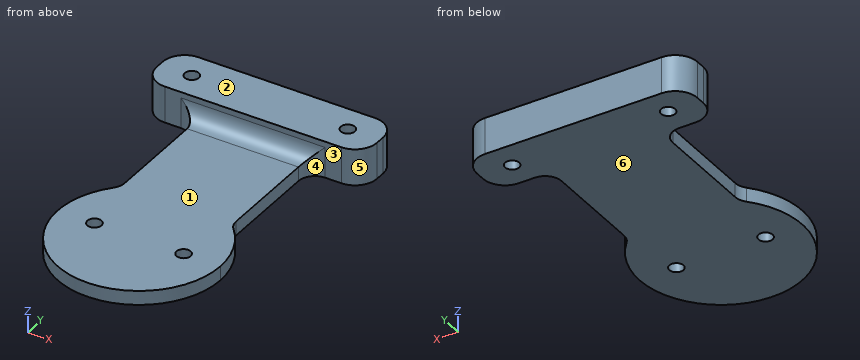
```python
from build123d import *

# Parameters (mm, degrees)
F1_DEPTH = 3.175
F3_DEPTH = 5
F4_R     = 3.6792614691
F5_R     = 1.5875
F6_DEPTH = 24.13
F7_DEPTH = 25.4
F8_R     = 4.9056819587


with BuildPart() as f1:
    # F0 (on Top) → F1 (new body)
    with BuildSketch(Plane.XY):
        with BuildLine():
            ThreePointArc((-12.4973059814, 13.2996181602), (0, 18.25), (12.4973059814, 13.2996181602))
            Line((12.4973059814, 13.2996181602), (12.4973059814, 40.75))
            Line((12.4973059814, 40.75), (24.7193473562, 40.75))
            Line((24.7193473562, 40.75), (24.7193473562, 52.75))
            Line((24.7193473562, 52.75), (-24.7193473562, 52.75))
            Line((-24.7193473562, 52.75), (-24.7193473562, 40.75))
            Line((-24.7193473562, 40.75), (-12.4973059814, 40.75))
            Line((-12.4973059814, 40.75), (-12.4973059814, 13.2996181602))
        make_face()
        with BuildLine():
            ThreePointArc((-12.4973059814, 13.2996181602), (-7.2452282862, -16.7501990161), (18.25, 0))
            ThreePointArc((18.25, 0), (16.7501990161, 7.2452282862), (12.4973059814, 13.2996181602))
            ThreePointArc((12.4973059814, 13.2996181602), (0, 18.25), (-12.4973059814, 13.2996181602))
        make_face()
    extrude(amount=F1_DEPTH)

    # F2 (on face) → F3 (join)
    with BuildSketch(Plane.XY.offset(3.175)):
        Polygon((-24.7193473562, 40.75), (-12.4973059814, 40.75), (12.4973059814, 40.75), (24.7193473562, 40.75), (24.7193473562, 52.75), (-24.7193473562, 52.75), align=None)
    extrude(amount=F3_DEPTH)

    # F4
    f4_edges = [f1.edges().sort_by_distance(p)[0] for p in [
        (12.497306, 13.299618, 1.5875),
        (-12.497306, 13.299618, 1.5875),
        (12.497306, 40.75, 1.5875),
        (0, 40.75, 3.175),
        (-12.497306, 40.75, 1.5875),
    ]]
    fillet(f4_edges, radius=F4_R)

    # F5 (on face) → F6 (cut)
    with BuildSketch(Plane.XY.offset(3.175)):
        with Locations((-10, 0)):
            Circle(F5_R)
        with Locations((10, 0)):
            Circle(F5_R)
        with Locations((17.5, 46.75)):
            Circle(F5_R)
        with Locations((-17.5, 46.75)):
            Circle(F5_R)
    extrude(amount=F6_DEPTH, mode=Mode.SUBTRACT)

    # F5 (on face) → F7 (cut)
    with BuildSketch(Plane.XY.offset(3.175)):
        with Locations((-10, 0)):
            Circle(F5_R)
        with Locations((10, 0)):
            Circle(F5_R)
        with Locations((17.5, 46.75)):
            Circle(F5_R)
        with Locations((-17.5, 46.75)):
            Circle(F5_R)
    extrude(amount=-F7_DEPTH, mode=Mode.SUBTRACT)

    # F8
    f8_edges = [f1.edges().sort_by_distance(p)[0] for p in [
        (24.719347, 40.75, 4.0875),
        (24.719347, 52.75, 4.0875),
        (-24.719347, 52.75, 4.0875),
        (-24.719347, 40.75, 4.0875),
    ]]
    fillet(f8_edges, radius=F8_R)


solid = f1.part
```
Could you check a few things on this model? Use its own coordinates, in mm. Face numbers are marked on the shaded views. A direction names the side the tool comes from. Round coordinates to 2 decimals unless told otherwise and drop trailing zeros. Loops run counter-clockwise (first coordinate to the right, second up) from the corner with the lowest first, then second, coordinate; pieces in that order, holes last. Notation, with made-up numbers: (3, 88) -> (30, 88) arc R10 ccw to (30, 107) -> close; hole circle Ø8 at (86.5, 24). An arc over 180 degrees is marked (long way). One line per question, with ' | ' between items.
(1) If we section it at A-A on z = 1: Count the separate pieces of the cut face and the enclosed holes in it, and give its area (3 significant figures).
Model answer:
separate pieces: 1 | enclosed holes: 4 | area: 2,190 mm^2
(2) For pin 1 Ø2 at (x, y) = (11.5, 31) entering from +Z (3 decimals); pin 2 Ø4 at (x, y) = (15, 23.5) entering from -Z; pin 3 Ø1 at (y, z) = (9, 3.5) entering from -X; pin 4 Ø1.6 at (y, z) = (26.5, 1) entering from -X, each with a flat end and sliding along its axis, tell me the tip position at first contact or that it passes through.
Model answer:
pin 1: stops at z = 3.175 | pin 2: passes through | pin 3: stops at x = -16.09 | pin 4: stops at x = -12.5
(3) If we section it at B-B on y = 46.75: List the corners of the cut face in (x, z) for me (1 decimal).
Model answer:
outline: (-24.7, 0) -> (-19.1, 0) -> (-19.1, 8.2) -> (-24.7, 8.2) -> close; (-15.9, 0) -> (15.9, 0) -> (15.9, 8.2) -> (-15.9, 8.2) -> close; (19.1, 0) -> (24.7, 0) -> (24.7, 8.2) -> (19.1, 8.2) -> close
(4) For the marked faces 1, 2 and 3, which set-ups out of +Z, -Z, +X, -X, +Y, -Y let a thin tool reach every point of the face, with its end or its side?
Model answer:
face 1: +Z, +X, -X, -Y | face 2: +Z, +X, -X, +Y, -Y | face 3: +Z
(5) If I drill on probe 1 along X at (y, z) = (46.75, 6.75); probe 2 along Y at (x, z) = (17.5, 5); probe 3 along Y at (x, z) = (-6, 7), over which ranges is the centre line in solid material (lowest first)?
Model answer:
probe 1: x = -24.72 to -19.09, -15.91 to 15.91, 19.09 to 24.72 | probe 2: y = 40.75 to 45.16, 48.34 to 52.75 | probe 3: y = 40.75 to 52.75
(6) Thinking about a two-plate mould opening in Y: for the marked faces 4, 5 and 6, which applies, released by +Y, released by -Y, zero draft, split by the parting line, or undercut?
Model answer:
face 4: undercut | face 5: released by -Y | face 6: zero draft
